Solid Edge part; units mm, degrees
sketch "Sketch1" plane through (0, 0, 0) normal (0, 0, 1) x (1, 0, 0)
  line L0 (-38.736, 0) -> (191.264, 0)
  line L1 (191.264, 0) -> (191.264, 300)
  line L2 (191.264, 300) -> (-38.736, 300)
  line L3 (-38.736, 300) -> (-38.736, 0)
  dimension "D1" = 38.736
  dimension "D2" = 38.736
extrude "Protrusion1" add sketch "Sketch1" along normal blind 10
hole "Hole_1" at (6.264, 285, 10) direction (0, 0, -1) diameter 7 end up to next
hole "Hole1" at (6.264, 255, 10) direction (0, 0, -1) diameter 7 end up to next
hole "Hole2" at (-23.736, 255, 10) direction (0, 0, -1) diameter 7 end up to next
hole "Hole3" at (-23.736, 45, 10) direction (0, 0, -1) diameter 7 end up to next
hole "Hole4" at (6.264, 45, 10) direction (0, 0, -1) diameter 7 end up to next
hole "Hole5" at (6.264, 15, 10) direction (0, 0, -1) diameter 7 end up to next
hole "Hole6" at (-23.736, 15, 10) direction (0, 0, -1) diameter 7 end up to next
hole "Hole7" at (-23.736, 285, 10) direction (0, 0, -1) diameter 7 end up to next
hole "Hole8" at (146.264, 45, 10) direction (0, 0, -1) diameter 7 end up to next
hole "Hole9" at (176.264, 45, 10) direction (0, 0, -1) diameter 7 end up to next
hole "Hole10" at (176.264, 15, 10) direction (0, 0, -1) diameter 7 end up to next
hole "Hole11" at (146.264, 15, 10) direction (0, 0, -1) diameter 7 end up to next
hole "Hole12" at (146.264, 285, 10) direction (0, 0, -1) diameter 7 end up to next
hole "Hole13" at (176.264, 285, 10) direction (0, 0, -1) diameter 7 end up to next
hole "Hole14" at (176.264, 255, 10) direction (0, 0, -1) diameter 7 end up to next
hole "Hole15" at (146.264, 255, 10) direction (0, 0, -1) diameter 7 end up to next
hole "Hole_30" at (14.264, 204, 0) direction (0, 0, 1) diameter 10 end up to next
hole "Hole16" at (-12.736, 73, 0) direction (0, 0, 1) diameter 10 end up to next
hole "Hole17" at (118.264, 46, 0) direction (0, 0, 1) diameter 10 end up to next
hole "Hole18" at (145.264, 177, 0) direction (0, 0, 1) diameter 10 end up to next
properties material "Aluminum, 6061-T6"
Work out the finished part from the listing and answer in its coordinate system (mm). Give positions to 0.01 mm unless a question says otherwise; leave off trailing zeros. Order: outer loops, then holes, each group sorted by start corner. A loop starts at its lowest first (then second) coordinate and runs counter-clockwise, first axis right, second up.
1. Section C-C, the plane y = 45 is taken. Determine the outline of the cut face in (x, z).
Result sheet:
outline: (-38.74, 0) - (-27.24, 0) - (-27.24, 10) - (-38.74, 10) - close; (-20.24, 0) - (2.76, 0) - (2.76, 10) - (-20.24, 10) - close; (9.76, 0) - (113.37, 0) - (113.37, 10) - (9.76, 10) - close; (123.16, 0) - (142.76, 0) - (142.76, 10) - (123.16, 10) - close; (149.76, 0) - (172.76, 0) - (172.76, 10) - (149.76, 10) - close; (179.76, 0) - (191.26, 0) - (191.26, 10) - (179.76, 10) - close
2. Straight lines are drawn through the part: L1, parallel to X at y = 15, z = 5.5; L2, parallel to X at y = 73, z = 3.25; L3, parallel to Y at x = 6, z = 6.75. For each, find the intervals that lie inside material, in ascending order.
Result sheet:
L1: x = -38.74 to -27.24, -20.24 to 2.76, 9.76 to 142.76, 149.76 to 172.76, 179.76 to 191.26
L2: x = -38.74 to -17.74, -7.74 to 191.26
L3: y = 0 to 11.51, 18.49 to 41.51, 48.49 to 251.51, 258.49 to 281.51, 288.49 to 300
3. Section B-B, the plane y = 204 is taken. Determine the outline of the cut face in (x, z), and give its area (3 significant figures).
Result sheet:
outline: (-38.74, 0) - (9.26, 0) - (9.26, 10) - (-38.74, 10) - close; (19.26, 0) - (191.26, 0) - (191.26, 10) - (19.26, 10) - close
area: 2,200 mm2
4. Section A-A, the plane y = 285 is taken. Determine the outline of the cut face in (x, z), and give its area (3 significant figures).
Result sheet:
outline: (-38.74, 0) - (-27.24, 0) - (-27.24, 10) - (-38.74, 10) - close; (-20.24, 0) - (2.76, 0) - (2.76, 10) - (-20.24, 10) - close; (9.76, 0) - (142.76, 0) - (142.76, 10) - (9.76, 10) - close; (149.76, 0) - (172.76, 0) - (172.76, 10) - (149.76, 10) - close; (179.76, 0) - (191.26, 0) - (191.26, 10) - (179.76, 10) - close
area: 2,020 mm2
5. This flat-tipped pin is pushed along its axis until it touches: P1, Ø4, axis at x = -23.736, y = 285, coming from the +Z side. Where does it stop, or does it pass through?
Result sheet:
P1: passes through
6. The mould has two halves that part along Y. Classify faces 1 (the flat face through (191.264, 148, 5)), 2 (the flat face through (75, 0, 5)), 3 (the cylindrical face through (6.418, 48.497, 5.07)): released by +Y, released by -Y, zero draft, split by the parting line, or undercut.
Result sheet:
face 1: zero draft
face 2: released by -Y
face 3: undercut
